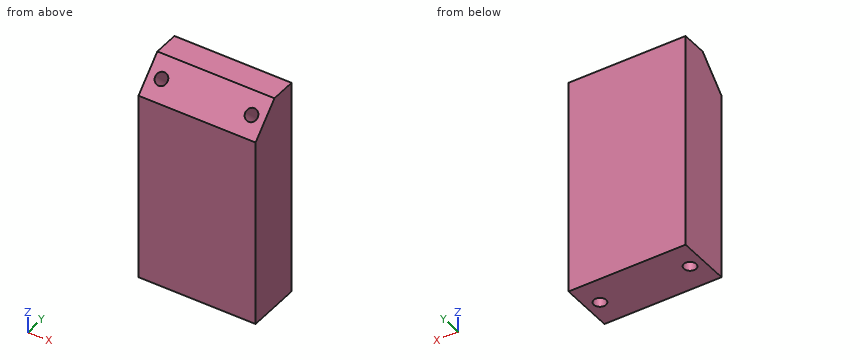
```python
from build123d import *

# Parameters (mm, degrees)
F0_W     = 82.55
F0_H     = 38.1
F1_DEPTH = 153.3652
F2_SIZE2 = 20.0152
F2_SIZE  = 20.0152
F4_D     = 8.7376
F4_DEPTH = 25.4
F4_TIP   = 2.6250398724
F6_D     = 8.7376
F6_DEPTH = 25.4
F6_TIP   = 2.6250398724


with BuildPart() as f1:
    # F0 (on Top) → F1 (new body)
    with BuildSketch(Plane.XY):
        with Locations((41.275, 19.05)):
            Rectangle(F0_W, F0_H)
    extrude(amount=F1_DEPTH)

    # F2
    f2_edges = [f1.edges().sort_by_distance(p)[0] for p in [
        (41.275, 0, 153.3652),
    ]]
    chamfer(f2_edges, length=F2_SIZE, length2=F2_SIZE2)

    # F4
    with Locations(Plane(origin=(0, -66.675, 66.675), x_dir=(1, 0, 0), z_dir=(0, -0.7071067812, 0.7071067812))):
        with Locations((9.525, 108.4455765648), (73.025, 108.4455765648)):
            Hole(F4_D / 2, depth=F4_DEPTH)
            with Locations((0, 0, -(F4_DEPTH + F4_TIP / 2))):  # 118° drill point
                Cone(0, F4_D / 2, F4_TIP, mode=Mode.SUBTRACT)

    # F6
    with Locations(Plane(origin=(0, 0, 0), x_dir=(1, 0, 0), z_dir=(0, 0, -1))):
        with Locations((9.525, -19.05), (73.025, -19.05)):
            Hole(F6_D / 2, depth=F6_DEPTH)
            with Locations((0, 0, -(F6_DEPTH + F6_TIP / 2))):  # 118° drill point
                Cone(0, F6_D / 2, F6_TIP, mode=Mode.SUBTRACT)


solid = f1.part
```
Input: part model. Units: mm. Frame: model coordinates. Round coordinates to 2 decimals unless told otherwise and drop trailing zeros. Write each loop counter-clockwise with the first axis right and the second up, starting at its lowest first coordinate (ties: lowest second). Pieces come first, ordered by that corner, then holes. Notation, with made-up numbers: (37.25, -2) - (83.25, -2) arc R10 ccw to (83.25, 14) - close; hole circle Ø8 at (51, 29.5). An arc over 180 degrees is marked (long way). Write item = value, one per line.
(1) Section query A-A on z = 12. Output: boundary loops of the cut face in (x, y) (3 decimals), then the cut area to 3 significant figures.
Geometry check:
outline = (0, 0) - (82.55, 0) - (82.55, 38.1) - (0, 38.1) - close; hole circle Ø8.738 at (9.525, 19.05); hole circle Ø8.738 at (73.025, 19.05)
area = 3,030 mm^2
(2) Section query C-C on y = 4. Output: boundary loops of the cut face in (x, z).
Geometry check:
outline = (0, 0) - (82.55, 0) - (82.55, 137.35) - (0, 137.35) - close
(3) Material intervals for probe 1 along X at (y, z) = (19.05, 5.5); probe 2 along Z at (x, y) = (7.5, 20.5); probe 3 along Y at (x, z) = (75, 22.5), sorted ascending.
Geometry check:
probe_1 = 0 to 5.16, 13.89 to 68.66, 77.39 to 82.55
probe_2 = 26.53 to 127.39, 138.34 to 153.37
probe_3 = 0 to 15.15, 22.95 to 38.1
(4) Section query B-B on x = 44. Output: boundary loops of the cut face in (y, z), then the cut area to 3 significant figures.
Geometry check:
outline = (0, 0) - (38.1, 0) - (38.1, 153.37) - (20.02, 153.37) - (0, 133.35) - close
area = 5,640 mm^2
